Geometry: see drawing. Coordinates: mm, zero at the bounding-box minimum. A direction names the side the tool comes from. Give positions to 0.01 mm unless a question says otherwise; leave off trailing zeros. Write each loop counter-clockwise with the first axis right and the second up, starting at its lowest first coordinate (ties: lowest second). Pieces come first, ordered by that corner, then holes. Notation, with made-up numbers: (16, -33) - (49, -33) arc R31 cw to (49, 3) - close; hole circle Ø5 at (12.25, -19.5). An arc over 180 degrees is marked (long way). Return JSON: item names as keys, results as strings.
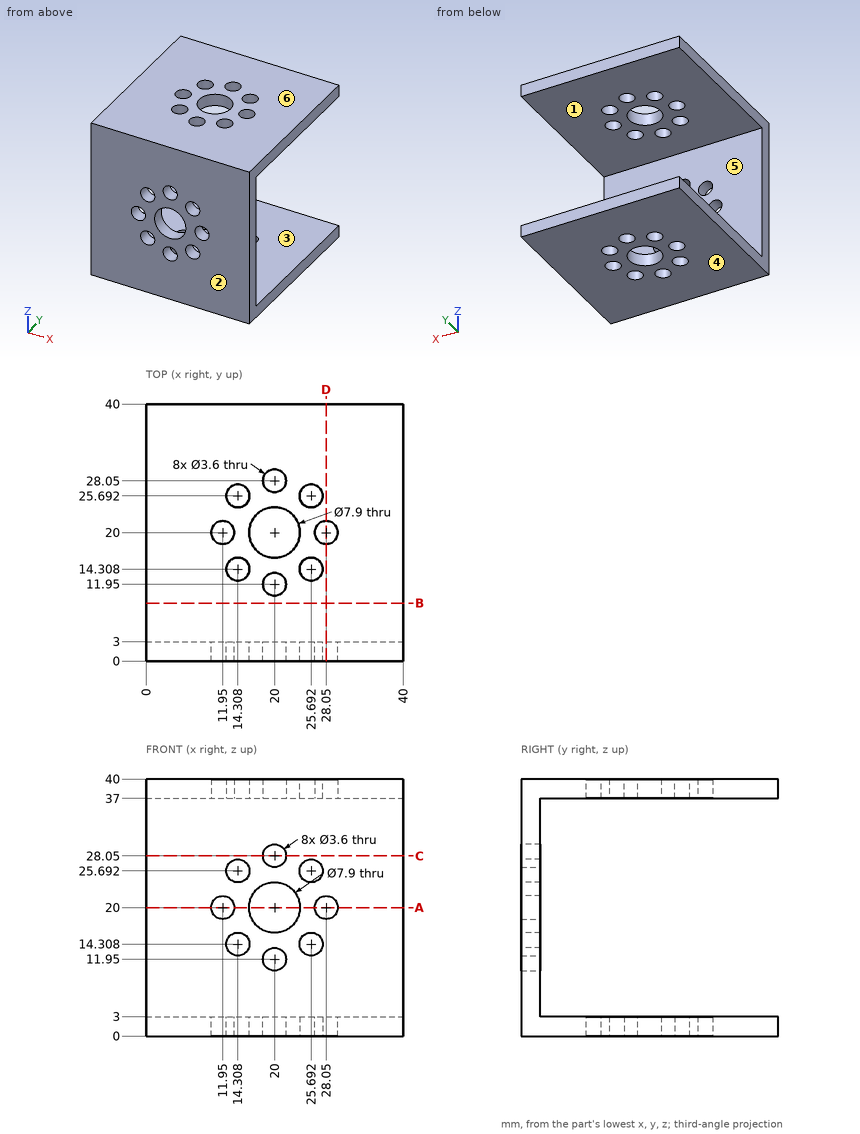
Q1. Set-up query: the marked faces 1 and 2. Return all of +Z, -Z, +X, -X, +Y, -Y with unobstructed straight access to the full face (end or side cutting, diameter ignored); none if empty.
Answer key:
{"face 1": "+X, -X, +Y", "face 2": "+Z, -Z, +X, -X, -Y"}
Q2. Section query D-D, the plane x = 28.05. Return the cut outline in (y, z), plus the area to 3 significant figures.
Answer key:
{"outline": "(0, 0) - (18.2, 0) - (18.2, 3) - (3, 3) - (3, 18.2) - (0, 18.2) - close; (0, 21.8) - (3, 21.8) - (3, 37) - (18.2, 37) - (18.2, 40) - (0, 40) - close; (21.8, 0) - (40, 0) - (40, 3) - (21.8, 3) - close; (21.8, 37) - (40, 37) - (40, 40) - (21.8, 40) - close", "area": "310 mm^2"}
Q3. Section query A-A, the plane z = 20. Return the cut outline in (x, y), plus the area to 3 significant figures.
Answer key:
{"outline": "(0, 0) - (10.15, 0) - (10.15, 3) - (0, 3) - close; (13.75, 0) - (16.05, 0) - (16.05, 3) - (13.75, 3) - close; (23.95, 0) - (26.25, 0) - (26.25, 3) - (23.95, 3) - close; (29.85, 0) - (40, 0) - (40, 3) - (29.85, 3) - close", "area": "74.7 mm^2"}
Q4. Pin query (flat end, axial travel): P1, Ø3, axis at x = 25.69, y = 25.69, coming from the -Z side; P2, Ø6, axis at x = 14.31, z = 14.31, coming from the +Y side. Return the tip coordinate at first contact, or that it passes through.
Answer key:
{"P1": "passes through", "P2": "stops at y = 3"}
Q5. Mould query, pull axis Z, two halves, no side actions, for the marked faces 3, 4, 5 and 6. Classes: pulls with the +Z half, pulls with the -Z half, needs draft (parallel to the pull), parting line crosses it, or undercut.
Answer key:
{"face 3": "undercut", "face 4": "pulls with the -Z half", "face 5": "undercut", "face 6": "pulls with the +Z half"}
Q6. Material intervals for probe 1 along Y at (x, z) = (20, 38.7); probe 2 along Z at (x, y) = (33.5, 37.5); probe 3 along Y at (x, z) = (20.5, 26), sorted ascending. Write a range as [from, to].
Answer key:
{"probe 1": "y = [0, 10.15], [13.75, 16.05], [23.95, 26.25], [29.85, 40]", "probe 2": "z = [0, 3], [37, 40]", "probe 3": "y = [0, 3]"}
Q7. Section query B-B, the plane y = 9. Return the cut outline in (x, z), plus the area to 3 significant figures.
Answer key:
{"outline": "(0, 0) - (40, 0) - (40, 3) - (0, 3) - close; (0, 37) - (40, 37) - (40, 40) - (0, 40) - close", "area": "240 mm^2"}
Q8. Section query C-C, the plane z = 28.05. Return the cut outline in (x, y), plus the area to 3 significant figures.
Answer key:
{"outline": "(0, 0) - (18.2, 0) - (18.2, 3) - (0, 3) - close; (21.8, 0) - (40, 0) - (40, 3) - (21.8, 3) - close", "area": "109 mm^2"}
